from build123d import *

# Parameters (mm, degrees)
F0_W     = 12.5222
F0_H     = 114.3
F1_DEPTH = 10.16
F3_DEPTH = 25.4
F4_W     = 12.5222
F4_H     = 12.7
F5_DEPTH = 22.86


with BuildPart() as f1:
    # F0 (on Top) → F1 (new body)
    with BuildSketch(Plane.XY):
        with Locations((-43.899023, -13.46517)):
            Rectangle(F0_W, F0_H)
    extrude(amount=F1_DEPTH)

    # F2 (on face) → F3 (cut)
    with BuildSketch(Plane.YZ.offset(-37.637923)):
        with BuildLine():
            ThreePointArc((-70.61517, 5.08), (-13.521586, 8.889373), (43.68483, 10.16))
            Line((43.68483, 10.16), (-70.61517, 10.16))
            Line((-70.61517, 10.16), (-70.61517, 5.08))
        make_face()
    extrude(amount=-F3_DEPTH, mode=Mode.SUBTRACT)

    # F4 (on face) → F5 (join)
    with BuildSketch(Plane(origin=(0, 0, 0), x_dir=(1, 0, 0), z_dir=(0, 0, -1))):
        with Locations((-43.899023, 64.26517)):
            Rectangle(F4_W, F4_H)
    extrude(amount=F5_DEPTH)


solid = f1.part
The model under review builds one solid part; all positions refer to its coordinate system, in mm. A direction names the side the tool comes from. Give positions to 0.01 mm unless a question says otherwise; leave off trailing zeros. Write each loop counter-clockwise with the first axis right and the second up, starting at its lowest first coordinate (ties: lowest second). Pieces come first, ordered by that corner, then holes. Notation, with made-up numbers: M 87.5,-26.75 L 102.5,-26.75 A21 cw 102.5,10.25 Z; hole C -18,8 d4. An arc over 180 degrees is marked long. One line per question, with ' | ' between items. Start each with the question number.
Item 1: For faces 4 (the flat face through (-44, 43.685, 5)), 5 (the flat face through (-44, -6, 0)), list the 3-axis set-ups (+Z, -Z, +X, -X, +Y, -Y) from which the entire face can be reached by the end or side of a thin tool; tool diameter is ignored.
Item 2: Wall thickness on line 1 (Y direction, x = -45.75, z = -8); line 2 (Z direction, x = -43, y = 24.5); line 3 (Z direction, x = -46.75, y = -58.5): over which ranges is each line inside the solid? List them lowest first. Write a range as from..to.
Item 3: For pin 1 (4 mm diameter, centred on x = -41, y = -48, fed in from -Z), flat-tipped, find the tip position at first contact; note if it passes through.
Item 4: We need section C-C on y = -32.5. Write out the cut boundary in (x, z), plus the area to 3 significant figures.
Item 5: We need section A-A on x = -41.5. Write out the cut boundary in (y, z), plus the area to 3 significant figures.
Item 6: We need section B-B on z = -15. Write out the cut boundary in (x, y).
Item 7: Draft analysis for pull direction Z (two halves, no side actions). For faces 1 (the flat face through (-44, -64, -22.86)), 2 (the flat face through (-37.638, -22, 4)), 3 (the cylindrical face through (-43.811, -14.322, 8.854)), state which applies: released by +Z, released by -Z, zero draft, split by the parting line, or undercut.
Results found:
1) face 4: +Z, -Z, +X, -X, +Y | face 5: -Z, +X, -X, +Y
2) line 1: y = -70.62..-57.92 | line 2: z = 0..10.02 | line 3: z = -22.86..6.1
3) pin 1: stops at z = 0
4) outline: M -50.16,0 L -37.64,0 L -37.64,7.91 L -50.16,7.91 Z | area: 99.0 mm2
5) outline: M -70.62,-22.86 L -57.92,-22.86 L -57.92,0 L 43.68,0 L 43.68,10.16 A1288.42 ccw -70.62,5.08 Z | area: 1,260 mm2
6) outline: M -50.16,-70.62 L -37.64,-70.62 L -37.64,-57.92 L -50.16,-57.92 Z
7) face 1: released by -Z | face 2: zero draft | face 3: released by +Z
